For this review, take the finished solid that the model builds, in its own axes (mm). A direction names the side the tool comes from. Coordinates: 2 decimals unless noted, no trailing zeros. Write each loop counter-clockwise with the first axis right and the second up, starting at its lowest first coordinate (ties: lowest second). Pieces come first, ordered by that corner, then holes.
1) We need section A-A on x = 7.5. Write out the cut boundary in (y, z).
2) Insertion check: P1, Ø1.5, axis at x = -13.5, y = -3.5, coming from the +Z side. The pin has a flat end and moves straight along its axis. Give the tip position at first contact, or say it passes through.
3) We need section C-C on z = 50. Write out the cut boundary in (x, y), then the cut area to 3 significant figures.
4) We need section B-B on y = -4.5. Write out the cut boundary in (x, z).
5) To check wall thickness, follow line 1 along Z through (x, y) = (0, -6.25); line 2 along Z through (x, y) = (3, -3.25); line 3 along Z through (x, y) = (9.5, -6.5). State the ranges of each line that lie inside material, in increasing order.
6) Mouldability with a two-part tool opening along X and no side actions: class faces 1 (the face through (-20, -5, -6)), 2 (the face through (10, -5, 80)), 3 (the face through (0, -5, -100)) as pulls with the +X half, pulls with the -X half, needs draft (parallel to the pull), parting line crosses it, or undercut.
7) For faces 4 (the face through (1, -5, 40)), 5 (the face through (0, -5, 100)), list the 3-axis set-ups (+Z, -Z, +X, -X, +Y, -Y) from which the entire face can be reached by the end or side of a thin tool; tool diameter is ignored.
from build123d import *

# Parameters (mm, degrees)
F0_W     = 40
F0_H     = 200
F0_W_2   = 5
F0_H_2   = 10
F0_R     = 2.5
F0_W_3   = 20
F0_H_3   = 20
F1_DEPTH = 10
F2_R     = 10


with BuildPart() as f1:
    # F0 (on Front) → F1 (new body)
    with BuildSketch(Plane.XZ):
        Rectangle(F0_W, F0_H)
        with Locations((-13.5, 50)):
            Rectangle(F0_W_2, F0_H_2, mode=Mode.SUBTRACT)
        with Locations((1.5, 35)):
            Rectangle(F0_W_2, F0_H_2, mode=Mode.SUBTRACT)
        with Locations((0, 50)):
            Circle(F0_R, mode=Mode.SUBTRACT)
        with Locations((0, 80.0469)):
            Rectangle(F0_W_3, F0_H_3, mode=Mode.SUBTRACT)
    extrude(amount=F1_DEPTH)

    # F2
    f2_edges = [f1.edges().sort_by_distance(p)[0] for p in [
        (20, -5, 100),
        (-20, -5, 100),
    ]]
    fillet(f2_edges, radius=F2_R)


solid = f1.part
Result:
1. outline: (-10, -100) - (0, -100) - (0, 70.05) - (-10, 70.05) - close; (-10, 90.05) - (0, 90.05) - (0, 100) - (-10, 100) - close
2. P1: stops at z = 99.61
3. outline: (-20, -10) - (-16, -10) - (-16, 0) - (-20, 0) - close; (-11, -10) - (-2.5, -10) - (-2.5, 0) - (-11, 0) - close; (2.5, -10) - (20, -10) - (20, 0) - (2.5, 0) - close
3. area: 300 mm2
4. outline: (-20, -100) - (20, -100) - (20, 90) arc R10 ccw to (10, 100) - (-10, 100) arc R10 ccw to (-20, 90) - close; hole (-16, 45) - (-11, 45) - (-11, 55) - (-16, 55) - close; hole (-10, 70.05) - (10, 70.05) - (10, 90.05) - (-10, 90.05) - close; hole circle Ø5 at (0, 50); hole (-1, 30) - (4, 30) - (4, 40) - (-1, 40) - close
5. line 1: z = -100 to 30, 40 to 47.5, 52.5 to 70.05, 90.05 to 100
5. line 2: z = -100 to 30, 40 to 70.05, 90.05 to 100
5. line 3: z = -100 to 70.05, 90.05 to 100
6. face 1: pulls with the -X half
6. face 2: undercut
6. face 3: needs draft
7. face 4: +Y, -Y
7. face 5: +Z, +X, -X, +Y, -Y
